Geometry: final body of the model. Coordinates: model frame, mm. A direction names the side the tool comes from. Round coordinates to 2 decimals unless told otherwise and drop trailing zeros. Write each loop counter-clockwise with the first axis right and the second up, starting at its lowest first coordinate (ties: lowest second). Pieces come first, ordered by that corner, then holes. Notation, with made-up numbers: (54, -0.75) -> (85, -0.75) arc R24 cw to (85, 26.25) -> close; hole circle Ø7 at (78.25, 82). An arc over 180 degrees is marked (long way). Use one line per item in the form item = value. Start each with the question number.
1. Reachability of faces 5 (the face through (15, -3.414, 26)), 6 (the face through (15, -6, -19.615)), 7 (the face through (15, 20.986, -22)) from +Z, -Z, +X, -X, +Y, -Y: full face, straight path, thin tool, end or side. Return the list, or none.
2. Pin query (flat end, axial travel): pin 1 Ø10 at (x, y) = (4, -5.5) entering from +Z; pin 2 Ø4.5 at (x, z) = (15, -22) entering from +Y; pin 3 Ø3 at (x, y) = (11, 19) entering from -Z. Return the tip coordinate at first contact, or that it passes through.
3. Cut plane B-B, the plane y = 9.5. Return the cut outline in (x, z), plus the area to 3 significant figures.
4. Line query: L1, parallel to Z at x = 10.33, y = 12.5; L2, parallel to Z at x = 19.83, y = 17.5; L3, parallel to X at y = 8.5, z = 0. Output: solid intervals per line, ascending.
5. Cut plane A-A, the plane x = 7.5. Return the cut outline in (y, z).
6. Draft query along Y for faces 1 (the face through (12.52, -28.11, -14.62)), 2 (the face through (15, -0.556, -26)), 3 (the face through (25.4, 8, -24)), 4 (the face through (15, 20.986, 22)). Return one class per face: pulls with the +Y half, pulls with the -Y half, needs draft (parallel to the pull), parting line crosses it, or undercut.
7. Cut plane C-C, the plane z = 0. Return the cut outline in (x, y).
8. Cut plane D-D, the plane y = 16. Return the cut outline in (x, z).
```python
from build123d import *

# Parameters (mm, degrees)
SKETCH1_R           = 31.6865
BOSS_EXTRUDE1_DEPTH = 25.4
CUT_EXTRUDE1_START  = -20.32
CUT_EXTRUDE1_DEPTH  = 20.32
SKETCH5_R           = 0.508
CUT_EXTRUDE2_DEPTH  = 12.7
SKETCH6_R           = 0.508
CUT_EXTRUDE3_DEPTH  = 3.556


# Read off the part's stored shape, not the designer's step: Cut-Extrude1
with BuildPart() as part:
    # Sketch1 → Boss-Extrude1 (new body)
    with BuildSketch(Plane(origin=(0, 0, 0), x_dir=(0, 0, -1), z_dir=(1, 0, 0))):
        Circle(SKETCH1_R)
    extrude(amount=BOSS_EXTRUDE1_DEPTH)

    # Cut-Extrude1 outline → Cut-Extrude1 (cut)
    with BuildSketch(Plane(origin=(25.4, 0, 0), x_dir=(0, 0, -1), z_dir=(1, 0, 0)).offset(CUT_EXTRUDE1_START)):
        with BuildLine():
            Line((31.681621585, -0.556), (19.614864522, -0.556))
            Line((19.614864522, -0.556), (19.614864522, 20.9865))
            Line((19.614864522, 20.9865), (23.740284329, 20.9865))
            ThreePointArc((23.740284329, 20.9865), (0, 31.6865), (-23.740284329, 20.9865))
            Line((-23.740284329, 20.9865), (-20.785135478, 20.9865))
            Line((-20.785135478, 20.9865), (-20.785135478, -0.556))
            Line((-20.785135478, -0.556), (-31.681621585, -0.556))
            ThreePointArc((-31.681621585, -0.556), (-31.624152047, -1.986778691), (-31.50209993, -3.4135))
            Line((-31.50209993, -3.4135), (-20.785135478, -3.4135))
            Line((-20.785135478, -3.4135), (-20.785135478, -9.415012817))
            Line((-20.785135478, -9.415012817), (19.614864522, -9.415012817))
            Line((19.614864522, -9.415012817), (19.614864522, -3.4135))
            Line((19.614864522, -3.4135), (31.50209993, -3.4135))
            ThreePointArc((31.50209993, -3.4135), (31.624152047, -1.986778691), (31.681621585, -0.556))
        make_face()
    extrude(amount=CUT_EXTRUDE1_DEPTH, mode=Mode.SUBTRACT)

    # Sketch5 → Cut-Extrude2 (cut)
    with BuildSketch(Plane(origin=(0, 20.9865, 0), x_dir=(1, 0, 0), z_dir=(0, 1, 0))):
        with Locations(Location((10.33, -24.932573059, 0), (0, 0, 270))):
            Circle(SKETCH5_R)
        with Locations(Location((19.83, -24.932573059, 0), (0, 0, 270))):
            Circle(SKETCH5_R)
        with Locations(Location((10.33, 23.762302103, 0), (0, 0, 270))):
            Circle(SKETCH5_R)
        with Locations(Location((19.83, 23.762302103, 0), (0, 0, 270))):
            Circle(SKETCH5_R)
    extrude(amount=-CUT_EXTRUDE2_DEPTH, mode=Mode.SUBTRACT)

    # Sketch6 → Cut-Extrude3 (cut)
    with BuildSketch(Plane.ZY):
        with Locations((-1.539927539, 19.940627452)):
            Circle(SKETCH6_R)
    extrude(amount=-CUT_EXTRUDE3_DEPTH, mode=Mode.SUBTRACT)


solid = part.part
```
Outcome:
q1.face_5 = +Z, -Z, +X
q1.face_6 = +X, +Y
q1.face_7 = +Z, -Z, +X, +Y
q2.pin_1 = 31.68
q2.pin_2 = 20.99
q2.pin_3 = -26.42
q3.outline = (0, -30.23) -> (25.4, -30.23) -> (25.4, -19.61) -> (5.08, -19.61) -> (5.08, 20.79) -> (25.4, 20.79) -> (25.4, 30.23) -> (0, 30.23) -> close; hole circle Ø1.02 at (10.33, -23.76); hole circle Ø1.02 at (10.33, 24.93); hole circle Ø1.02 at (19.83, -23.76); hole circle Ø1.02 at (19.83, 24.93)
q3.area = 711 mm^2
q4.L1 = -29.12 to -24.27, -23.25 to -19.61, 20.79 to 24.42, 25.44 to 29.12
q4.L2 = -26.42 to -24.27, -23.25 to -19.61, 20.79 to 24.42, 25.44 to 26.42
q4.L3 = 0 to 5.08
q5.outline = (-9.42, -19.61) -> (-9.42, 20.79) -> (-3.41, 20.79) -> (-3.41, 31.5) arc R31.69 ccw to (-3.41, -31.5) -> (-3.41, -19.61) -> close; (-0.56, -31.68) arc R31.69 ccw to (20.99, -23.74) -> (20.99, -19.61) -> (-0.56, -19.61) -> close; (-0.56, 20.79) -> (20.99, 20.79) -> (20.99, 23.74) arc R31.69 ccw to (-0.56, 31.68) -> close
q6.face_1 = parting line crosses it
q6.face_2 = undercut
q6.face_3 = needs draft
q6.face_4 = pulls with the +Y half
q7.outline = (0, -31.69) -> (25.4, -31.69) -> (25.4, -9.42) -> (5.08, -9.42) -> (5.08, 31.69) -> (0, 31.69) -> close
q8.outline = (0, -27.35) -> (25.4, -27.35) -> (25.4, -19.61) -> (5.08, -19.61) -> (5.08, 20.79) -> (25.4, 20.79) -> (25.4, 27.35) -> (0, 27.35) -> close; hole circle Ø1.02 at (10.33, -23.76); hole circle Ø1.02 at (10.33, 24.93); hole circle Ø1.02 at (19.83, -23.76); hole circle Ø1.02 at (19.83, 24.93)
